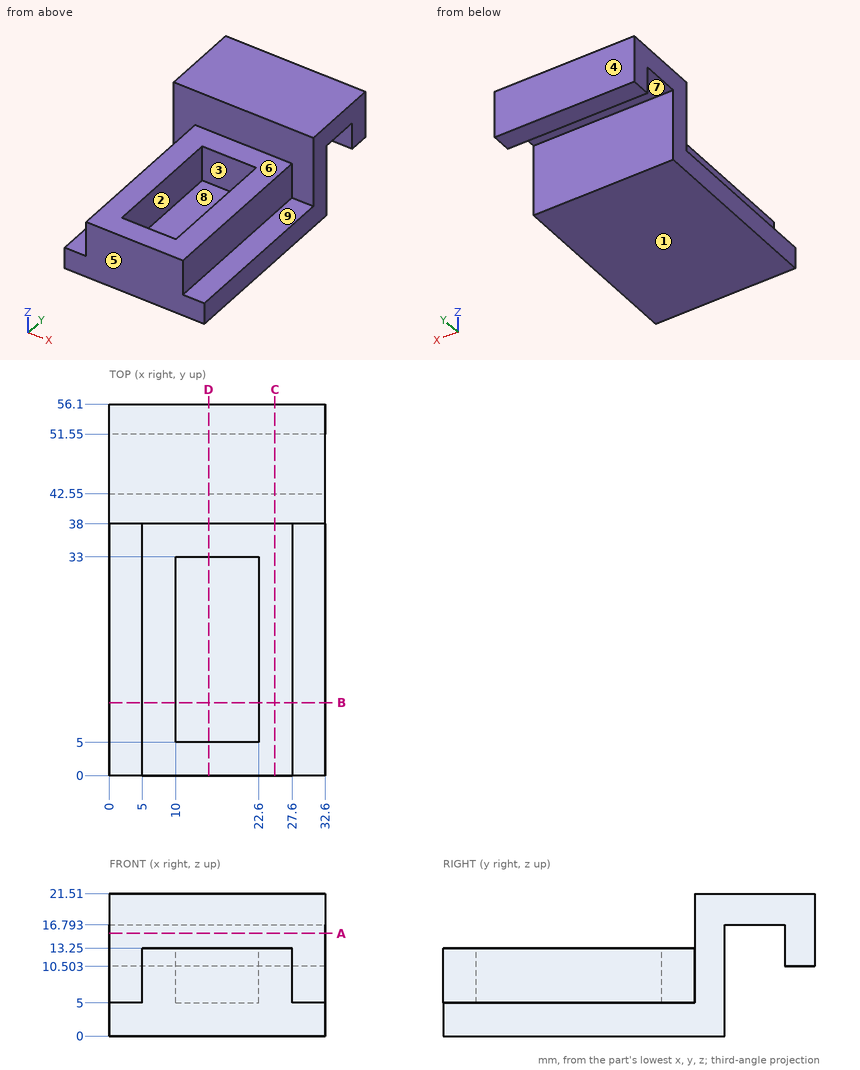
Print and shaded views of the part. All mm, measured from the part's lowest x, y and z. A direction names the side the tool comes from. Give positions to 0.01 mm unless a question says otherwise; leave off trailing zeros. Loops run counter-clockwise (first coordinate to the right, second up) from the corner with the lowest first, then second, coordinate; pieces in that order, holes last.
1) Saw through at D-D (x = 15). Write the cut outline in (y, z), plus the area to 3 significant figures.
2) Saw through at B-B (y = 11). Write the cut outline in (x, z).
3) Saw through at A-A (z = 15.5). Write the cut outline in (x, y), plus the area to 3 significant figures.
4) Wall check: line 1 (Y direction, x = 11.5, z = 10); line 2 (Y direction, x = 21, z = 14); line 3 (X direction, y = 9, z = 11.5). Give the ranges that are in metal, low to high.
5) Flat gauge pins, fed straight in: pin 1 Ø6.5 at (x, z) = (15.5, 10) entering from -Y; pin 2 Ø2.5 at (y, z) = (25.5, 8.5) entering from +X; pin 3 Ø1.5 at (x, z) = (10.5, 8) entering from +Y; pin 4 Ø4 at (x, y) = (21.5, 14.5) entering from +Z. Where does each tip first touch, or does it go through?
6) Pull direction Y, two halves, no side cores. Call the marked faces 1, 2, 3 and 4: +Y half, -Y half, draft (parallel to the pull), parting line (faces both ways), or undercut.
7) Tool access for the marked faces 5, 6, 7, 8 and 9: list every direction of +Z, -Z, +X, -X, +Y, -Y with a clear straight run to the whole face (end or side of a thin tool).
8) Saw through at C-C (x = 25). Write the cut outline in (y, z).
Answer block:
1. outline: (0, 0) - (42.55, 0) - (42.55, 16.79) - (51.55, 16.79) - (51.55, 10.5) - (56.1, 10.5) - (56.1, 21.51) - (38, 21.51) - (38, 13.25) - (33, 13.25) - (33, 5) - (5, 5) - (5, 13.25) - (0, 13.25) - close
1. area: 463 mm2
2. outline: (0, 0) - (32.6, 0) - (32.6, 5) - (27.6, 5) - (27.6, 13.25) - (22.6, 13.25) - (22.6, 5) - (10, 5) - (10, 13.25) - (5, 13.25) - (5, 5) - (0, 5) - close
3. outline: (0, 38) - (32.6, 38) - (32.6, 42.55) - (0, 42.55) - close; (0, 51.55) - (32.6, 51.55) - (32.6, 56.1) - (0, 56.1) - close
3. area: 297 mm2
4. line 1: y = 0 to 5, 33 to 42.55
4. line 2: y = 38 to 42.55, 51.55 to 56.1
4. line 3: x = 5 to 10, 22.6 to 27.6
5. pin 1: stops at y = 0
5. pin 2: stops at x = 27.6
5. pin 3: stops at y = 42.55
5. pin 4: stops at z = 13.25
6. face 1: draft
6. face 2: undercut
6. face 3: undercut
6. face 4: +Y half
7. face 5: +Z, -Z, +X, -X, -Y
7. face 6: +Z, +X, -X, -Y
7. face 7: -Z, +X, -X
7. face 8: +Z
7. face 9: +Z, +X, -Y
8. outline: (0, 0) - (42.55, 0) - (42.55, 16.79) - (51.55, 16.79) - (51.55, 10.5) - (56.1, 10.5) - (56.1, 21.51) - (38, 21.51) - (38, 13.25) - (0, 13.25) - close
